from build123d import *

# Parameters (mm, degrees)
SKETCH1_W           = 60
SKETCH1_H           = 270
BOSS_EXTRUDE1_DEPTH = 5
SKETCH2_W           = 50
SKETCH2_H           = 50
BOSS_EXTRUDE3_DEPTH = 2
LPATTERN1_COUNT     = 5
LPATTERN1_PITCH     = 52
SKETCH3_W           = 52
SKETCH3_H           = 51.9
BOSS_EXTRUDE8_DEPTH = 25
LPATTERN5_COUNT     = 5
LPATTERN5_PITCH     = 52


with BuildPart() as part:
    # Sketch1 → Boss-Extrude1 (new body)
    with BuildSketch(Plane(origin=(0, 0, 0), x_dir=(1, 0, 0), z_dir=(0, 1, 0))):
        Rectangle(SKETCH1_W, SKETCH1_H)
    extrude(amount=BOSS_EXTRUDE1_DEPTH)

    # Sketch2 → Boss-Extrude3 (add)
    with BuildSketch(Plane(origin=(0, 5, 0), x_dir=(1, 0, 0), z_dir=(0, 1, 0))):
        with Locations((0, -105)):
            Rectangle(SKETCH2_W, SKETCH2_H)
    boss_extrude3 = extrude(amount=BOSS_EXTRUDE3_DEPTH)

    # LPattern1: Boss-Extrude3 ×5
    with Locations(*[(0, 0, -i * LPATTERN1_PITCH) for i in range(1, LPATTERN1_COUNT)]):
        add(boss_extrude3)

    # Sketch3 → Boss-Extrude8 (add)
    with BuildSketch(Plane(origin=(0, 7, 0), x_dir=(1, 0, 0), z_dir=(0, 1, 0))):
        with Locations((0, -105.05)):
            Rectangle(SKETCH3_W, SKETCH3_H)
    boss_extrude8 = extrude(amount=BOSS_EXTRUDE8_DEPTH)

    # LPattern5: Boss-Extrude8 ×5
    with Locations(*[(0, 0, -i * LPATTERN5_PITCH) for i in range(1, LPATTERN5_COUNT)]):
        add(boss_extrude8)


solid = part.part
Source: CAD feature listing. Evaluate the final solid. Frame: model axes, mm. A direction names the side the tool comes from. Give positions to 0.01 mm unless a question says otherwise; leave off trailing zeros. Loops run counter-clockwise (first coordinate to the right, second up) from the corner with the lowest first, then second, coordinate; pieces in that order, holes last. Notation, with made-up numbers: (-3.75, 36) -> (31.25, 36) arc R26 ccw to (31.25, 70) -> close; hole circle Ø2 at (74.5, 44). An arc over 180 degrees is marked (long way). Use a Markdown table: item, result. Add a question column.
1) Line query: line 1 along Y through (x, z) = (-25.5, -39.5); line 2 along X through (y, z) = (27.5, 85.5). Output: solid intervals per line, ascending. Write a range as [from, to].
2) First-contact query: pin 1 (1.6 mm diameter, centred on y = 5.5, z = 5.5, fed in from +X); pin 2 (7.5 mm diameter, centred on y = 25, z = -49.5, fed in from +X); pin 3 (2 mm diameter, centred on x = -15, y = 13.5, fed in from -Z); pin 4 (1.6 mm diameter, centred on y = 6, z = -93.5, fed in from -X). Flat tips, straight axial feed; report the tip coordinate or a pass-through.
3) Pull-direction query (Y, two-part tool) for faces 5 (the face through (0, 32, -103)), 6 (the face through (30, 2, 2)), 7 (the face through (-25.2, 7, 41.4)); classes: +Y half, -Y half, draft (parallel to the pull), parting line (faces both ways), or undercut.
4) Section query B-B, the plane z = 89. Return the cut outline in (x, y).
5) Section query A-A, the plane y = 14. Return the cut outline in (x, z).
6) Reachability of faces 1 (the face through (0, 19, 131)), 2 (the face through (0, 2, 135)), 3 (the face through (26, 19, -103)), 4 (the face through (-26, 19, -103)) from +Z, -Z, +X, -X, +Y, -Y: full face, straight path, thin tool, end or side. Return the list, or none.
Numbers:
| question | item | result |
|---|---|---|
| 1 | line 1 | y = [0, 5], [7, 32] |
| 1 | line 2 | x = [-26, 26] |
| 2 | pin 1 | stops at x = 30 |
| 2 | pin 2 | stops at x = 26 |
| 2 | pin 3 | stops at z = -128.9 |
| 2 | pin 4 | stops at x = -25 |
| 3 | face 5 | +Y half |
| 3 | face 6 | draft |
| 3 | face 7 | undercut |
| 4 | outline | (-30, 0) -> (30, 0) -> (30, 5) -> (25, 5) -> (25, 7) -> (26, 7) -> (26, 32) -> (-26, 32) -> (-26, 7) -> (-25, 7) -> (-25, 5) -> (-30, 5) -> close |
| 5 | outline | (-26, -128.9) -> (26, -128.9) -> (26, -77) -> (-26, -77) -> close; (-26, -76.9) -> (26, -76.9) -> (26, -25) -> (-26, -25) -> close; (-26, -24.9) -> (26, -24.9) -> (26, 27) -> (-26, 27) -> close; (-26, 27.1) -> (26, 27.1) -> (26, 79) -> (-26, 79) -> close; (-26, 79.1) -> (26, 79.1) -> (26, 131) -> (-26, 131) -> close |
| 6 | face 1 | +Z, +X, -X, +Y |
| 6 | face 2 | +Z, +X, -X, +Y, -Y |
| 6 | face 3 | +Z, -Z, +X, +Y |
| 6 | face 4 | +Z, -Z, -X, +Y |
